```python
from build123d import *

# Parameters (mm, degrees)
F0_R     = 25
F1_DEPTH = 10
F2_W     = 38.7
F2_H     = 10.2
F3_DEPTH = 11
F4_W     = 10.2
F4_H     = 1.3916883618
F5_DEPTH = 2
F6_W     = 10.2
F6_H     = 1.392
F7_DEPTH = 2
F9_DEPTH = 25


# Not quite as in the source:
# - a fillet or chamfer that OpenCascade refuses, or shapes differently, is made with other operations: its cross-section is extruded or revolved along the edge and cut away or added


with BuildPart() as f1:
    # F0 (on Top) → F1 (new body)
    with BuildSketch(Plane.XY):
        Circle(F0_R)
    extrude(amount=F1_DEPTH)

    # F2 (on face) → F3 (cut)
    with BuildSketch(Plane.XY.offset(10)):
        with Locations((-0.05, -0.05)):
            Rectangle(F2_W, F2_H)
    extrude(amount=-F3_DEPTH, mode=Mode.SUBTRACT)

    # F4 (on face) → F5 (join)
    with BuildSketch(Plane(origin=(19.3, 0, 0), x_dir=(0, -1, 0), z_dir=(-1, 0, 0))):
        with Locations((0.05, 0.6958441809)):
            Rectangle(F4_W, F4_H)
    extrude(amount=F5_DEPTH)

    # F6 (on face) → F7 (join)
    with BuildSketch(Plane.YZ.offset(-19.4)):
        with Locations((-0.05, 0.696)):
            Rectangle(F6_W, F6_H)
    extrude(amount=F7_DEPTH)

    # F8 (on face) → F9 (cut)
    with BuildSketch(Plane(origin=(0, -5.15, 0), x_dir=(-1, 0, 0), z_dir=(0, 1, 0))):
        with BuildLine():
            Line((-8.5235216661, 0), (8.5235216661, 0))
            ThreePointArc((8.5235216661, 0), (0, 8.5235216661), (-8.5235216661, 0))
        make_face()
    extrude(amount=-F9_DEPTH, mode=Mode.SUBTRACT)

    # F10: fillet of radius 2 on 1 edges, made by hand

    # F10_s1 → F10_t2 (revolve, cut)
    with BuildSketch(Plane.XZ):
        with BuildLine():
            ThreePointArc((25, 8), (24.4142135624, 9.4142135624), (23, 10))
            Line((23, 10), (25, 10))
            Line((25, 10), (25, 8))
        make_face()
    revolve(axis=Axis((0, 0, 10), (0, 0, 1)), mode=Mode.SUBTRACT)


solid = f1.part
```
Here's how the part is built. I have some questions about the finished solid (model axes, mm). A direction names the side the tool comes from. Round coordinates to 2 decimals unless told otherwise and drop trailing zeros. Order: outer loops, then holes, each group sorted by start corner. A loop starts at its lowest first (then second) coordinate and runs counter-clockwise, first axis right, second up. Notation, with made-up numbers: M -13,80.5 L 6,80.5 A26 cw 6,110.5 Z; hole C 78.25,50.5 d1. An arc over 180 degrees is marked long. Answer in a Markdown table with one row per item.
Item 1: If I drill on L1, parallel to Y at x = -14.5, z = 3.75; L2, parallel to X at y = 4, z = 2.25; L3, parallel to X at y = -11.5, z = 3.25, over which ranges is the centre line in solid material (lowest first)? Write a range as from..to.
A:
| item | result |
|---|---|
| L1 | y = -20.37..-5.15, 5.05..20.37 |
| L2 | x = -24.68..-19.4, 19.3..24.68 |
| L3 | x = -22.2..-7.88, 7.88..22.2 |
Item 2: Imagine slicing it at B-B, the plane x = 0. Write out the boundary of the cut face in (y, z), and give its area (3 significant figures).
A:
| item | result |
|---|---|
| outline | M -24.93,8.52 L -5.15,8.52 L -5.15,10 L -23,10 A2 ccw Z; M 5.05,0 L 25,0 L 25,8 A2 ccw 23,10 L 5.05,10 Z |
| area | 227 mm2 |
Item 3: I'm going to push flat-ended pins straight in: pin 1 (5 mm diameter, centred on y = 6, z = 2.5, fed in from -X); pin 2 (3 mm diameter, centred on x = 4, z = 3, fed in from -Y); pin 3 (1.1 mm diameter, centred on y = 1.5, z = 0.5, fed in from +X). Where does each tip first touch, or does it pass through?
A:
| item | result |
|---|---|
| pin 1 | stops at x = -24.75 |
| pin 2 | stops at y = 5.05 |
| pin 3 | stops at x = 24.98 |
Item 4: Imagine slicing it at A-A, the plane y = 0. Write out the boundary of the cut face in (x, z).
A:
| item | result |
|---|---|
| outline | M -25,0 L -17.4,0 L -17.4,1.39 L -19.4,1.39 L -19.4,10 L -23,10 A2 ccw -25,8 Z; M 17.3,0 L 25,0 L 25,8 A2 ccw 23,10 L 19.3,10 L 19.3,1.39 L 17.3,1.39 Z |
Item 5: Imagine slicing it at D-D, the plane z = 6. Write out the boundary of the cut face in (x, y).
A:
| item | result |
|---|---|
| outline | M -19.4,-5.15 L -19.4,5.05 L 19.3,5.05 L 19.3,-5.15 L 6.05,-5.15 L 6.05,-24.26 A25 ccw long -6.05,-24.26 L -6.05,-5.15 Z |
Item 6: Thinking about a two-plate mould opening in Y: for faces 4 (the face through (-17.4, 0, 1)), 5 (the face through (-0.3, 5.4, 10)), 6 (the face through (-0.3, -5.15, 9.5)), 7 (the face through (1.058, 24.978, 3.944)), which applies, +Y half, -Y half, draft (parallel to the pull), parting line (faces both ways), or undercut?
A:
| item | result |
|---|---|
| face 4 | undercut |
| face 5 | draft |
| face 6 | undercut |
| face 7 | parting line |
Item 7: For faces 1 (the face through (18, 0, 1.392)), 2 (the face through (-0.19, -14.9, 8.52)), 3 (the face through (17.3, 0, 1)), which set-ups out of +Z, -Z, +X, -X, +Y, -Y let a thin tool reach every point of the face, with its end or its side?
A:
| item | result |
|---|---|
| face 1 | +Z |
| face 2 | -Z, -Y |
| face 3 | +Z, -Z |
Item 8: Imagine slicing it at C-C, the plane z = 3. Write out the boundary of the cut face in (x, y), and give its area (3 significant figures).
A:
| item | result |
|---|---|
| outline | M -19.4,-5.15 L -19.4,5.05 L 19.3,5.05 L 19.3,-5.15 L 7.98,-5.15 L 7.98,-23.69 A25 ccw long -7.98,-23.69 L -7.98,-5.15 Z |
| area | 1,260 mm2 |
